```python
from build123d import *

# Parameters (mm, degrees)
F1_DEPTH = 50.8
F2_R     = 1.27
F3_R     = 5.08
F4_SIZE  = 0.635
F5_R     = 5.08


with BuildPart() as f1:
    # F0 (on Top) → F1 (new body, symmetric)
    with BuildSketch(Plane.XY):
        Polygon((25.423321, 6.35), (0, 76.2), (0, 6.35), (-14.25222, 6.35), (-14.25222, 0), (0, 0), (52.093321, 0), (52.093321, 19.05), (45.743321, 19.05), (45.743321, 6.35), align=None)
    extrude(amount=F1_DEPTH, both=True)

    # F2
    f2_edges = [f1.edges().sort_by_distance(p)[0] for p in [
        (0, 76.2, 0),
    ]]
    fillet(f2_edges, radius=F2_R)

    # F3
    f3_edges = [f1.edges().sort_by_distance(p)[0] for p in [
        (52.093321, 0, 0),
        (52.093321, 9.525, -50.8),
        (52.093321, 19.05, 0),
        (52.093321, 9.525, 50.8),
    ]]
    fillet(f3_edges, radius=F3_R)

    # F4
    f4_edges = [f1.edges().sort_by_distance(p)[0] for p in [
        (45.743321, 6.35, 0),
        (0, 6.35, 0),
    ]]
    chamfer(f4_edges, length=F4_SIZE)

    # F5
    f5_edges = [f1.edges().sort_by_distance(p)[0] for p in [
        (-14.25222, 6.35, 0),
    ]]
    fillet(f5_edges, radius=F5_R)


solid = f1.part
```
Model file for the job. Use its own axes, mm. A direction names the side the tool comes from. Round coordinates to 2 decimals unless told otherwise and drop trailing zeros. Write each loop counter-clockwise with the first axis right and the second up, starting at its lowest first coordinate (ties: lowest second). Pieces come first, ordered by that corner, then holes. Notation, with made-up numbers: (-26, -18.75) - (15, -18.75) arc R21 cw to (15, 4.25) - close; hole circle Ø4 at (-22.5, -34.5). An arc over 180 degrees is marked (long way). One line per item, written item: value.
(1) Wall check: probe 1 along Y at (x, z) = (45, -11); probe 2 along X at (y, z) = (15, 31). Give the ranges that are in metal, low to high.
Values follow:
probe 1: y = 0 to 6.35
probe 2: x = 0 to 22.27, 45.74 to 51.99
(2) 3-axis set-ups, long thin cutter, end or side, ignore diameter. For faces 4 (the cylindrical face through (50.645, 1.528, 0.711)), 5 (the flat face through (0, 38, 1)), 6 (the flat face through (35, 6.35, 1)): which of +Z, -Z, +X, -X, +Y, -Y reach the whole face in a straight line?
Values follow:
face 4: +Z, -Z, +X, -Y
face 5: +Z, -Z, -X, +Y
face 6: +Z, -Z, +Y
(3) Two-plate mould, pull along X, no slides. Class faces 1 (the flat face through (16, 0, 1)), 2 (the flat face through (45.743, 13, 1)), 3 (the cylindrical face through (1.07, 70.25, 0.71)): pulls with the +X half, pulls with the -X half, needs draft (parallel to the pull), parting line crosses it, or undercut.
Values follow:
face 1: needs draft
face 2: undercut
face 3: parting line crosses it
(4) Drop flat-ended pins along their axis: P1, Ø1.5, axis at y = 28.5, z = 40.5, coming from the -X side; P2, Ø6, axis at x = 39, z = 17.5, coming from the +Y side; P3, Ø7, axis at x = -4, z = -25, coming from the +Y side (3 decimals). Give the stop position or say it passes through.
Values follow:
P1: stops at x = 0
P2: stops at y = 6.35
P3: stops at y = 6.485
(5) Cut at A-A, the plane y = 15.5. Give the cut face in (x, z).
Values follow:
outline: (0, -50.8) - (22.09, -50.8) - (22.09, 50.8) - (0, 50.8) - close; (45.74, -50.8) - (47.01, -50.8) arc R5.08 ccw to (51.86, -47.25) - (51.86, 47.25) arc R5.08 ccw to (47.01, 50.8) - (45.74, 50.8) - close
(6) Cut at D-D, the plane y = 63.5. Give the cut face in (x, z), plus the area to 3 significant figures.
Values follow:
outline: (0, -50.8) - (4.62, -50.8) - (4.62, 50.8) - (0, 50.8) - close
area: 470 mm²
(7) Cut at C-C, the plane x = 37.5. Give the cut face in (y, z), plus the area to 3 significant figures.
Values follow:
outline: (0, -50.8) - (6.35, -50.8) - (6.35, 50.8) - (0, 50.8) - close
area: 645 mm²
(8) Cut at B-B, the plane z = 23. Give the cut face in (x, y) (3 decimals).
Values follow:
outline: (-14.252, 0) - (47.013, 0) arc R5.08 ccw to (52.093, 5.08) - (52.093, 13.97) arc R5.08 ccw to (47.013, 19.05) - (45.743, 19.05) - (45.743, 6.985) - (45.108, 6.35) - (25.423, 6.35) - (2.463, 69.432) arc R1.27 ccw to (0, 68.997) - (0, 6.985) - (-0.635, 6.35) - (-9.172, 6.35) arc R5.08 ccw to (-14.252, 1.27) - close
